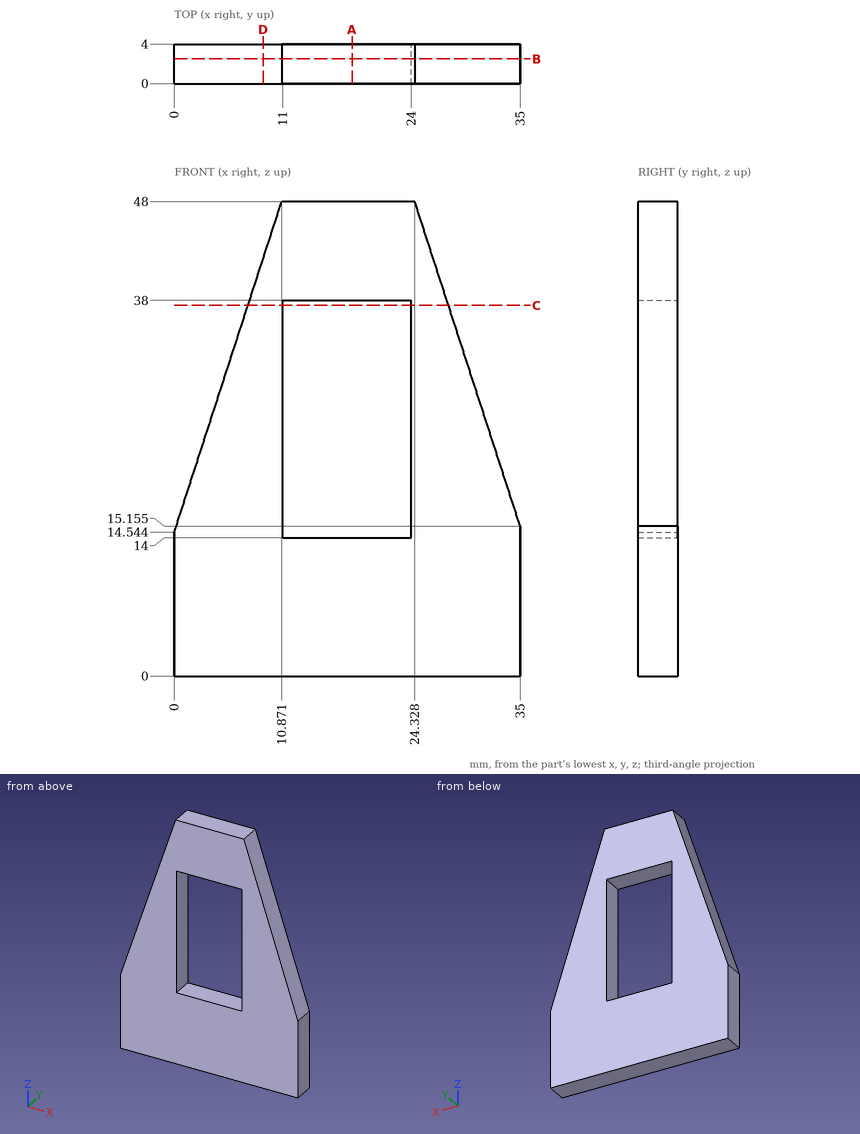
Drawing for the job (mm, zero at the part's lowest x, y, z). Round coordinates to 2 decimals unless told otherwise and drop trailing zeros. Write each loop counter-clockwise with the first axis right and the second up, starting at its lowest first coordinate (ties: lowest second). Pieces come first, ordered by that corner, then holes. Notation, with made-up numbers: M 21,55.5 L 69,55.5 A36 cw 69,92.5 Z; hole C 15,44 d5. An arc over 180 degrees is marked long. Answer in a Markdown table with one row per item.
1. Saw through at D-D (x = 9). List the corners of the cut face in (y, z), and give its area (3 significant figures).
Geometry check:
| item | result |
|---|---|
| outline | M 0,0 L 4,0 L 4,42.24 L 0,42.24 Z |
| area | 169 mm2 |
2. Saw through at C-C (z = 37.5). List the corners of the cut face in (x, y).
Geometry check:
| item | result |
|---|---|
| outline | M 7.46,0 L 11,0 L 11,4 L 7.46,4 Z; M 24,0 L 27.74,0 L 27.74,4 L 24,4 Z |
3. Saw through at A-A (x = 18). List the corners of the cut face in (y, z).
Geometry check:
| item | result |
|---|---|
| outline | M 0,0 L 4,0 L 4,14 L 0,14 Z; M 0,38 L 4,38 L 4,48 L 0,48 Z |
4. Probe L1, parallel to Z at x = 20.5, y = 3.2; L2, parallel to X at y = 1.2, z = 14.5; L3, parallel to X at y = 0.95, z = 36.5 (1 decimal). List the from-to ranges inside material, lowest first. Write a range as [from, to].
Geometry check:
| item | result |
|---|---|
| L1 | [0, 14], [38, 48] |
| L2 | [0, 11], [24, 35] |
| L3 | [7.1, 11], [24, 28.1] |
5. Flat gauge pins, fed straight in: P1, Ø1, axis at y = 2, z = 35, coming from the -X side (1 decimal); P2, Ø2, axis at y = 1, z = 17, coming from the +X side (1 decimal); P3, Ø6, axis at x = 28.5, z = 15, coming from the -Y side. Where does each tip first touch, or does it go through?
Geometry check:
| item | result |
|---|---|
| P1 | x = 6.5 |
| P2 | x = 34.7 |
| P3 | y = 0 |
6. Saw through at B-B (y = 2.5). List the corners of the cut face in (x, z) (1 decimal).
Geometry check:
| item | result |
|---|---|
| outline | M 0,0 L 35,0 L 35,15.2 L 24.3,48 L 10.9,48 L 0,14.5 Z; hole M 11,14 L 24,14 L 24,38 L 11,38 Z |
